Source: three-view drawing plus pictorial views. Frame: mm from the lowest corner of the part. A direction names the side the tool comes from. Round coordinates to 2 decimals unless told otherwise and drop trailing zeros. Loops run counter-clockwise (first coordinate to the right, second up) from the corner with the lowest first, then second, coordinate; pieces in that order, holes last. Notation, with made-up numbers: (16, 1.5) -> (33, 1.5) arc R23 cw to (33, 9.5) -> close; hole circle Ø11 at (35.25, -6.75). An arc over 180 degrees is marked (long way). Put each result on its own line as item: value. Start each with the question number.
1. Cut plane A-A (z = 4.5). Return the cut outline in (x, y).
2. Cut plane B-B (x = 25). Return the cut outline in (y, z), then the cut area to 3 significant figures.
3. Material intervals for L1, parallel to Y at x = 25, z = 3.5; L2, parallel to Z at x = 25.5, y = 9.75; L3, parallel to X at y = 8, z = 4.5, sorted ascending.
4. Set-up query: the marked faces 1 and 2. Return all of +Z, -Z, +X, -X, +Y, -Y with unobstructed straight access to the full face (end or side cutting, diameter ignored); none if empty.
5. Cut plane C-C (y = 12.25). Return the cut outline in (x, z), then the cut area to 3 significant figures.
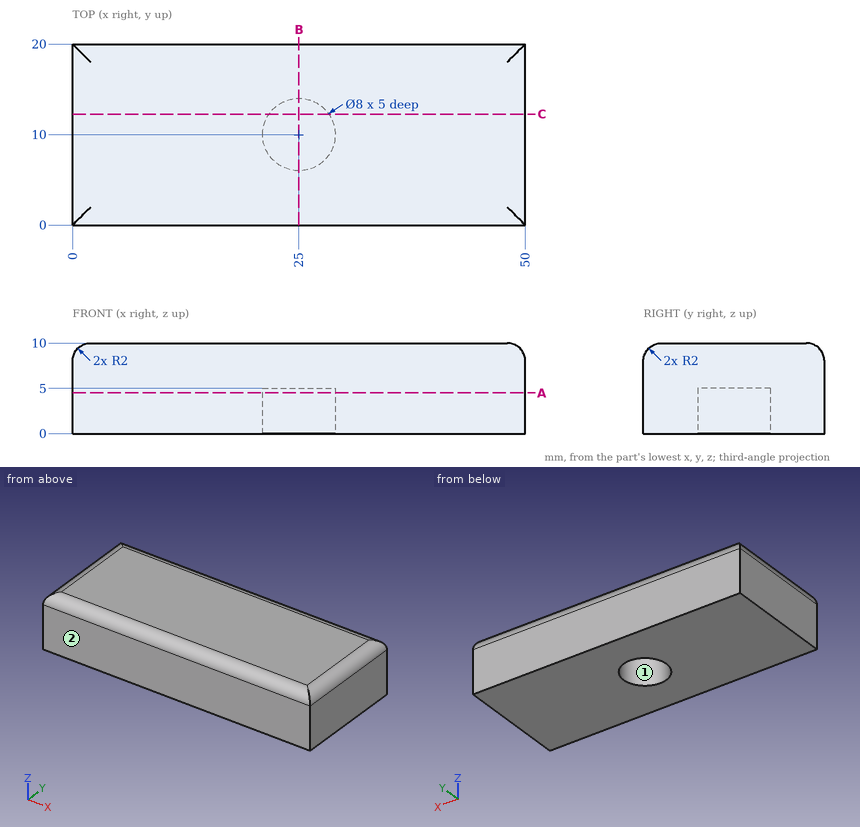
Solution:
1. outline: (0, 0) -> (50, 0) -> (50, 20) -> (0, 20) -> close; hole circle Ø8 at (25, 10)
2. outline: (0, 0) -> (6, 0) -> (6, 5) -> (14, 5) -> (14, 0) -> (20, 0) -> (20, 8) arc R2 ccw to (18, 10) -> (2, 10) arc R2 ccw to (0, 8) -> close
2. area: 158 mm^2
3. L1: y = 0 to 6, 14 to 20
3. L2: z = 5 to 10
3. L3: x = 0 to 21.54, 28.46 to 50
4. face 1: -Z
4. face 2: +Z, -Z, +X, -X, -Y
5. outline: (0, 0) -> (21.69, 0) -> (21.69, 5) -> (28.31, 5) -> (28.31, 0) -> (50, 0) -> (50, 8) arc R2 ccw to (48, 10) -> (2, 10) arc R2 ccw to (0, 8) -> close
5. area: 465 mm^2
